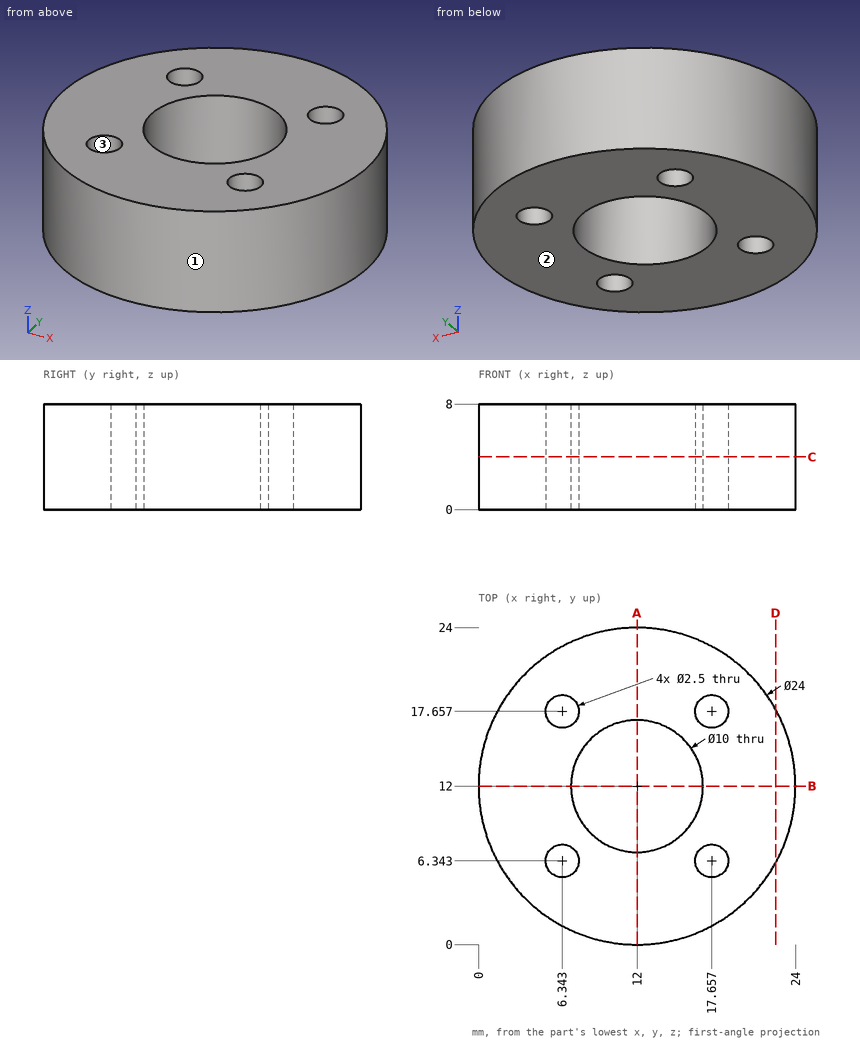
Here's the drawing with two shaded views (mm, measured from the low corner). I have some questions. Round coordinates to 2 decimals unless told otherwise and drop trailing zeros. Write each loop counter-clockwise with the first axis right and the second up, starting at its lowest first coordinate (ties: lowest second). Pieces come first, ordered by that corner, then holes. Notation, with made-up numbers: M 51.25,-29 L 82.25,-29 A20 ccw 82.25,-7 Z; hole C 3,29 d4. An arc over 180 degrees is marked long. Write each question's results on one line, items separated by ' | '. Start each with the question number.
1. Imagine slicing it at C-C on z = 4. List the corners of the cut face in (x, y) for me.
2. I'm going to push flat-ended pins straight in: pin 1 Ø4 at (x, y) = (6.34, 6.34) entering from -Z; pin 2 Ø3 at (y, z) = (16, 6.5) entering from +X; pin 3 Ø1.5 at (x, z) = (18.5, 1.5) entering from -Y; pin 4 Ø1.5 at (y, z) = (10, 5.5) entering from +X. Where does each tip first touch, or does it pass through?
3. I need wall thicknesses on L1, parallel to Y at x = 6.25, z = 1; L2, parallel to X at y = 17.25, z = 4.75 (1 decimal); L3, parallel to Y at x = 11.75, z = 0.75. Which ranges of each line are inside material? Lowest first, please. Write a range as from..to.
4. Imagine slicing it at D-D on x = 22.5. List the corners of the cut face in (y, z) for me.
5. Imagine slicing it at A-A on x = 12. List the corners of the cut face in (y, z) for me, and give its area (3 significant figures).
6. Thinking about a two-plate mould opening in X: for the marked faces 1, 2 and 3, which applies, +X half, -X half, draft (parallel to the pull), parting line (faces both ways), or undercut?
Result sheet:
1) outline: C 12,12 d24; hole C 6.34,6.34 d2.5; hole C 6.34,17.66 d2.5; hole C 12,12 d10; hole C 17.66,6.34 d2.5; hole C 17.66,17.66 d2.5
2) pin 1: stops at z = 0 | pin 2: stops at x = 23.74 | pin 3: stops at y = 1.47 | pin 4: stops at x = 23.93
3) L1: y = 1.47..5.1, 7.59..16.41, 18.9..22.53 | L2: x = 1.2..5.2, 7.5..16.5, 18.8..22.8 | L3: y = 0..7.01, 16.99..24
4) outline: M 6.19,0 L 17.81,0 L 17.81,8 L 6.19,8 Z
5) outline: M 0,0 L 7,0 L 7,8 L 0,8 Z; M 17,0 L 24,0 L 24,8 L 17,8 Z | area: 112 mm^2
6) face 1: parting line | face 2: draft | face 3: undercut
